from build123d import *

# Parameters (mm, degrees)
SKETCH1_W           = 28
SKETCH1_H           = 28
BOSS_EXTRUDE1_DEPTH = 203.2
SKETCH2_W           = 3.175
SKETCH2_H           = 28
CUT_EXTRUDE1_DEPTH  = 15
FILLET1_R           = 3.175


with BuildPart() as part:
    # Sketch1 → Boss-Extrude1 (new body)
    with BuildSketch(Plane(origin=(0, 0, 0), x_dir=(0, 0, -1), z_dir=(1, 0, 0))):
        Rectangle(SKETCH1_W, SKETCH1_H)
    extrude(amount=BOSS_EXTRUDE1_DEPTH)

    # Sketch2 → Cut-Extrude1 (cut)
    with BuildSketch(Plane(origin=(0, 14, 0), x_dir=(1, 0, 0), z_dir=(0, 1, 0))):
        with Locations((101.6, 0)):
            Rectangle(SKETCH2_W, SKETCH2_H)
    extrude(amount=-CUT_EXTRUDE1_DEPTH, mode=Mode.SUBTRACT)

    # Fillet1
    fillet1_edges = [part.edges().sort_by_distance(p)[0] for p in [
        (50.00625, 14, 14),
        (50.00625, 14, -14),
        (153.19375, 14, 14),
        (153.19375, 14, -14),
        (101.6, -14, -14),
        (101.6, -14, 14),
    ]]
    fillet(fillet1_edges, radius=FILLET1_R)


solid = part.part
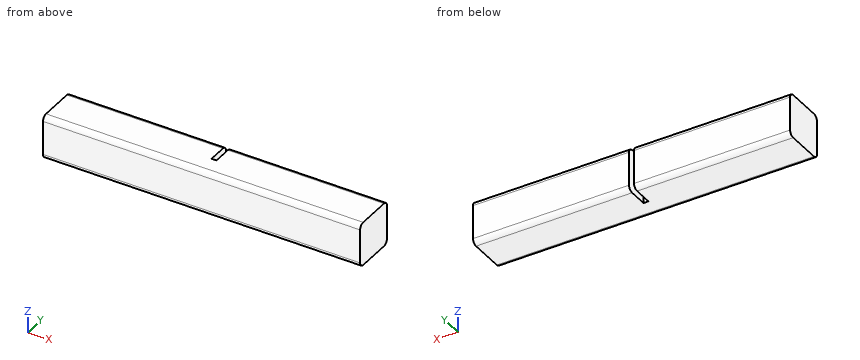
Design review of the part built by this model. Coordinates are the model's own, in mm. Coordinates: 2 decimals unless noted, no trailing zeros. Loops run counter-clockwise (first coordinate to the right, second up) from the corner with the lowest first, then second, coordinate; pieces in that order, holes last.
Item 1: Clearance check with a flat-ended pin moving along its axis: pin 1 (10 mm diameter, centred on y = -7, z = 0.5, fed in from -X). State where the tip first meets the part, or that it passes through.
Completed:
pin 1: stops at x = 0
Item 2: Add section A-A (y = 5.25). Write out the cut boundary in (x, z).
Completed:
outline: (0, -14) - (100.01, -14) - (100.01, 14) - (0, 14) - close; (103.19, -14) - (203.2, -14) - (203.2, 14) - (103.19, 14) - close
Item 3: Wall thickness on L1, parallel to X at y = 5, z = 6.5; L2, parallel to Z at x = 99, y = 11.5; L3, parallel to Z at x = 83.5, y = -12.5: over which ranges is each line inside the solid? List them lowest first.
Completed:
L1: x = 0 to 100.01, 103.19 to 203.2
L2: z = -13.93 to 13.93
L3: z = -13.52 to 13.52
